Geometry: final body of the model. Coordinates: model frame, mm. Round coordinates to 2 decimals unless told otherwise and drop trailing zeros. Order: outer loops, then holes, each group sorted by start corner. A loop starts at its lowest first (then second) coordinate and runs counter-clockwise, first axis right, second up. Notation, with made-up numbers: M 68.25,-6.75 L 86.25,-6.75 A18 cw 86.25,2.25 Z; hole C 68,56 d5. An arc over 180 degrees is marked long. Return JSON: item names as keys, results as strings. Group by question number.
Q1. Cut plane C-C on x = -57. Output: boundary loops of the cut face in (y, z), and give its area (3 significant figures).
Q2. Cut plane A-A on y = 100. Output: boundary loops of the cut face in (x, z), and give its area (3 significant figures).
Q3. Ray query, probe 1 along Y at (x, z) = (-42, 5.25); probe 2 along X at (y, z) = (106.5, 7.25); probe 3 along X at (y, z) = (87, 3.25). Return the intervals inside material, ascending.
Q4. Cut plane B-B on z = 2.75. Output: boundary loops of the cut face in (x, y), and give its area (3 significant figures).
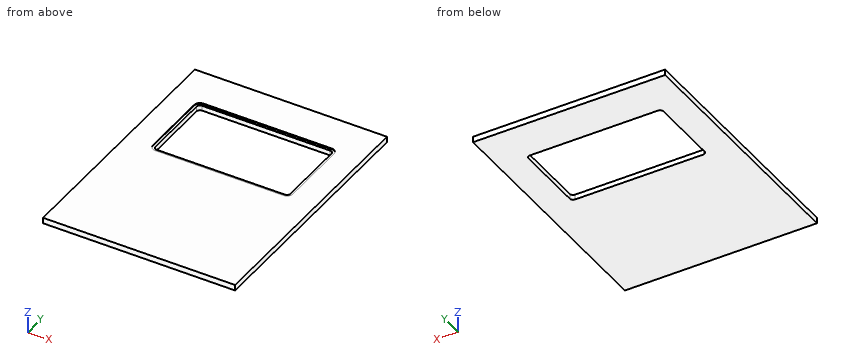
Autodesk Inventor part; units mm, degrees
ref_plane "YZ Plane" through (0, 0, 0) normal (1, 0, 0) x (0, 1, 0)
ref_plane "XZ Plane" through (0, 0, 0) normal (0, 1, 0) x (-1, 0, 0)
ref_plane "XY Plane" through (0, 0, 0) normal (0, 0, 1) x (1, 0, 0)
sketch "Sketch1" plane through (0, 0, 0) normal (0, 0, 1) x (1, 0, 0)
  line L0 (-132.5, 175) -> (132.5, 175)
  line L1 (132.5, 175) -> (132.5, -175)
  line L2 (132.5, -175) -> (-132.5, -175)
  line L3 (-132.5, -175) -> (-132.5, 175)
  point P0 (0, 0)
  dimension "d0" = 265
  dimension "d1" = 350
  dimension "d2" = 265
  dimension "d3" = 350
  dimension "d4" = 132.5
  dimension "d5" = 175
extrude "Extrusion1" add sketch "Sketch1" along normal blind 8
sketch "Sketch2" plane through (0, 0, 8) normal (0, 0, 1) x (1, 0, 0)
  line L0 (-96.5, 121) -> (96.5, 121)
  line L1 (96.5, 121) -> (96.5, 10)
  line L2 (96.5, 10) -> (-96.5, 10)
  line L3 (-96.5, 10) -> (-96.5, 121)
  point P0 (0, 0)
  dimension "d8" = 193
  dimension "d9" = 111
  dimension "d10" = 96.5
  dimension "d17" = 10
extrude "Extrusion2" cut sketch "Sketch2" against normal blind 1
fillet "Fillet1" radius 8 4 edges at (-96.5, 121, 7.5) (96.5, 121, 7.5) (96.5, 10, 7.5) (-96.5, 10, 7.5)
sketch "Sketch3" plane through (0, 0, 7) normal (0, 0, 1) x (1, 0, 0)
  arc A0 (-96.5, 18) -> (-88.5, 10) centre (-88.5, 18) ccw
  line L0 (88.5, 10) -> (-88.5, 10)
  arc A1 (88.5, 10) -> (96.5, 18) centre (88.5, 18) ccw
  line L1 (96.5, 113) -> (96.5, 18)
  arc A2 (96.5, 113) -> (88.5, 121) centre (88.5, 113) ccw
  line L2 (-88.5, 121) -> (88.5, 121)
  arc A3 (-88.5, 121) -> (-96.5, 113) centre (-88.5, 113) ccw
  line L3 (-96.5, 18) -> (-96.5, 113)
  arc A4 (-88.5, 117.5) -> (-93, 113) centre (-88.5, 113) ccw
  line L4 (-88.5, 117.5) -> (88.5, 117.5)
  arc A5 (93, 113) -> (88.5, 117.5) centre (88.5, 113) ccw
  line L5 (93, 113) -> (93, 18)
  arc A6 (88.5, 13.5) -> (93, 18) centre (88.5, 18) ccw
  line L6 (88.5, 13.5) -> (-88.5, 13.5)
  arc A7 (-93, 18) -> (-88.5, 13.5) centre (-88.5, 18) ccw
  line L7 (-93, 18) -> (-93, 113)
  point P0 (0, 0)
  dimension "d14" = 3.5
extrude "Extrusion3" cut sketch "Sketch3" against normal through all contours L4 A5 L5 A6 L6 A7 L7 A4
properties part number "masca raspberry"
Result sheet:
{
 "1": {"outline": "M -175,0 L 13.5,0 L 13.5,7 L 10,7 L 10,8 L -175,8 Z; M 117.5,0 L 175,0 L 175,8 L 121,8 L 121,7 L 117.5,7 Z", "area": "1,960 mm²"},
 "2": {"outline": "M -132.5,0 L -93,0 L -93,7 L -96.5,7 L -96.5,8 L -132.5,8 Z; M 93,0 L 132.5,0 L 132.5,8 L 96.5,8 L 96.5,7 L 93,7 Z", "area": "625 mm²"},
 "3": {"probe 1": "y = -175 to 13.5, 117.5 to 175", "probe 2": "x = -132.5 to -96.5, 96.5 to 132.5", "probe 3": "x = -132.5 to -93, 93 to 132.5"},
 "4": {"outline": "M -132.5,-175 L 132.5,-175 L 132.5,175 L -132.5,175 Z; hole M -93,18 A4.5 ccw -88.5,13.5 L 88.5,13.5 A4.5 ccw 93,18 L 93,113 A4.5 ccw 88.5,117.5 L -88.5,117.5 A4.5 ccw -93,113 Z", "area": "73,400 mm²"}
}
